For this review, take the finished solid that the model builds, in its own axes (mm). Face numbers are marked on the shaded views. A direction names the side the tool comes from. Give positions to 0.01 mm unless a question says otherwise; leave off trailing zeros. Loops run counter-clockwise (first coordinate to the right, second up) from the corner with the lowest first, then second, coordinate; pieces in that order, holes last. Notation, with made-up numbers: (25, 70.25) -> (83, 70.25) arc R24 cw to (83, 84.25) -> close; hole circle Ø5 at (18.5, 63). An arc over 180 degrees is marked (long way). Answer as CSV lines item,"result". Start each with the question number.
Item 1: For L1, parallel to X at y = 6.25, z = 0.85; L2, parallel to Y at x = -0.25, z = -0.5 (3 decimals); L3, parallel to X at y = -2.75, z = -0.4, list the stretches that pass through material, from the lowest coordinate up. Write a range as from..to.
Item 2: Add section B-B on z = 0.9. State the section outline as (x, y) points (3 decimals), plus the area to 3 significant figures.
Item 3: The part is to be moulded in two halves that separate along X. For the marked faces 1, 2 and 3, say which applies: +X half, -X half, draft (parallel to the pull), parting line (faces both ways), or undercut.
Item 4: Clearance check with a flat-ended pin moving along its axis: P1, Ø0.5, axis at x = 0, z = -0.5, coming from the +Y side (3 decimals). State where the tip first meets the part, or that it passes through.
Item 5: Add section C-C on y = -2.75. State the section outline as (x, z) points, plus the area to 3 significant figures.
Item 6: Machinability: for the marked faces 4 and 5, which of the approach directions +Z, -Z, +X, -X, +Y, -Y give a long, thin tool a straight path to every point of the face, cutting with its end or side? Answer none if there is none.
Item 7: Add section D-D on x = -1.25. State the section outline as (y, z) points (3 decimals), plus the area to 3 significant figures.
Item 8: Add section A-A on y = 2.5. State the section outline as (x, z) points.
```python
from build123d import *

# Parameters (mm, degrees)
BOSS_EXTRUDE1_DEPTH = 1.5


with BuildPart() as part:
    # Sketch1 → Boss-Extrude1 (new, symmetric)
    with BuildSketch(Plane.XY):
        with BuildLine():
            Line((8, -8.125), (-8, -8.125))
            Line((-8, -8.125), (-8, 8.125))
            Line((-8, 8.125), (-3, 8.125))
            Line((-3, 8.125), (-3, -1.625))
            ThreePointArc((-3, -1.625), (-2.267766953, -3.392766953), (-0.5, -4.125))
            Line((-0.5, -4.125), (0.5, -4.125))
            ThreePointArc((0.5, -4.125), (2.267766953, -3.392766953), (3, -1.625))
            Line((3, -1.625), (3, 8.125))
            Line((3, 8.125), (8, 8.125))
            Line((8, 8.125), (8, -8.125))
        make_face()
    extrude(amount=BOSS_EXTRUDE1_DEPTH, both=True)


solid = part.part
```
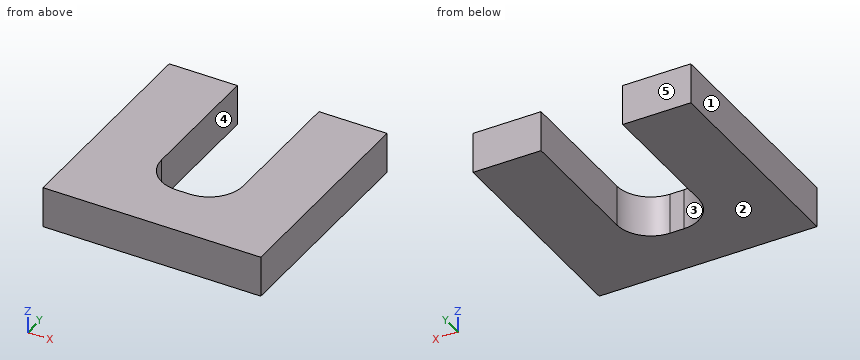
Computed values:
1,L1,"-8..-3, 3..8"
1,L2,"-8.125..-4.125"
1,L3,"-8..-2.73, 2.73..8"
2,outline,"(-8, -8.125) -> (8, -8.125) -> (8, 8.125) -> (3, 8.125) -> (3, -1.625) arc R2.5 cw to (0.5, -4.125) -> (-0.5, -4.125) arc R2.5 cw to (-3, -1.625) -> (-3, 8.125) -> (-8, 8.125) -> close"
2,area,"189 mm²"
3,face 1,"-X half"
3,face 2,"draft"
3,face 3,"undercut"
4,P1,"y = -4.125"
5,outline,"(-8, -1.5) -> (-2.73, -1.5) -> (-2.73, 1.5) -> (-8, 1.5) -> close; (2.73, -1.5) -> (8, -1.5) -> (8, 1.5) -> (2.73, 1.5) -> close"
5,area,"31.6 mm²"
6,face 4,"+Z, -Z, +Y"
6,face 5,"+Z, -Z, +X, -X, +Y"
7,outline,"(-8.125, -1.5) -> (-4.01, -1.5) -> (-4.01, 1.5) -> (-8.125, 1.5) -> close"
7,area,"12.3 mm²"
8,outline,"(-8, -1.5) -> (-3, -1.5) -> (-3, 1.5) -> (-8, 1.5) -> close; (3, -1.5) -> (8, -1.5) -> (8, 1.5) -> (3, 1.5) -> close"
